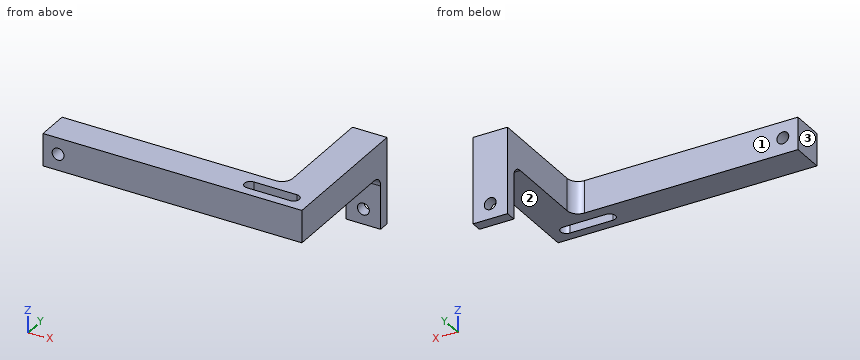
from build123d import *

# Parameters (mm, degrees)
BOSS_EXTRUDE1_DEPTH  = 15
SKETCH2_W            = 16
SKETCH2_H            = 5
BOSS_EXTRUDE2_DEPTH  = 40
CUT_EXTRUDE1_DEPTH   = 45
M5_CLEARANCE_HOLE1_D = 5.5
FILLET1_R            = 5


with BuildPart() as part:
    # Sketch1 → Boss-Extrude1 (new body)
    with BuildSketch(Plane.XY):
        Polygon((0, 0), (-120, 0), (-120, 15), (-16, 15), (-16, 62), (0, 62), align=None)
    extrude(amount=BOSS_EXTRUDE1_DEPTH)

    # Sketch2 → Boss-Extrude2 (add)
    with BuildSketch(Plane.XY.offset(15)):
        with Locations((-8, 64.5)):
            Rectangle(SKETCH2_W, SKETCH2_H)
    extrude(amount=-BOSS_EXTRUDE2_DEPTH)

    # Sketch3 → Cut-Extrude1 (cut)
    with BuildSketch(Plane.XY.offset(15)):
        with BuildLine():
            Line((-28, 9.7), (-8, 9.7))
            ThreePointArc((-8, 9.7), (-5.3, 7), (-8, 4.3))
            Line((-8, 4.3), (-28, 4.3))
            ThreePointArc((-28, 4.3), (-30.7, 7), (-28, 9.7))
        make_face()
    extrude(amount=-CUT_EXTRUDE1_DEPTH, mode=Mode.SUBTRACT)

    # M5 Clearance Hole1 (through all)
    with Locations(Plane(origin=(0, 67, 0), x_dir=(1, 0, 0), z_dir=(0, 1, 0))):
        with Locations((-8, 18), (-113, -7.5)):
            Hole(M5_CLEARANCE_HOLE1_D / 2)

    # Fillet1
    fillet1_edges = [part.edges().sort_by_distance(p)[0] for p in [
        (-16, 15, 7.5),
        (-8, 62, 0),
    ]]
    fillet(fillet1_edges, radius=FILLET1_R)


solid = part.part
Design review of the part built by this model. Coordinates are the model's own, in mm. Face numbers are marked on the shaded views. A direction names the side the tool comes from. Round coordinates to 2 decimals unless told otherwise and drop trailing zeros. Write each loop counter-clockwise with the first axis right and the second up, starting at its lowest first coordinate (ties: lowest second). Pieces come first, ordered by that corner, then holes. Notation, with made-up numbers: (56, -39.75) -> (68, -39.75) arc R17 cw to (68, -20.75) -> close; hole circle Ø8 at (87.5, 35). An arc over 180 degrees is marked (long way). One line per item, written item: value. Start each with the question number.
Q1. Tool access review of the marked faces 1, 2 and 3: name each direction out of +Z, -Z, +X, -X, +Y, -Y from which nothing blocks a thin tool from reaching the whole face with its end or side.
Q2. Add section D-D (z = -18). Give the boundary of the cut face in (x, y), then the cut area to 3 significant figures.
Q3. Add section B-B (y = 7). Give the boundary of the cut face in (x, z).
Q4. To check wall thickness, follow probe 1 along Z at (x, y) = (-8, 64); probe 2 along Y at (x, z) = (-12, 10.5); probe 3 along Z at (x, y) = (-113, 6.25). State the ranges of each line that lie inside material, in increasing order.
Q5. Add section A-A (z = 7.5). Give the boundary of the cut face in (x, y), then the cut area to 3 significant figures.
Q6. Add section C-C (x = -113). Give the boundary of the cut face in (y, z), then the cut area to 4 significant figures.
Q7. Insertion check: P1, Ø12, axis at x = -88, z = 10.5, coming from the +Y side; P2, Ø17.5, axis at x = -6, z = -15.5, coming from the -Y side. Each pin has a flat end and moves straight along its axis. Give the tip position at first contact, or say it passes through.
Response:
1. face 1: +Z, -Z, -X, +Y
1. face 2: -Z, +X, -X, -Y
1. face 3: +Z, -Z, -X, +Y, -Y
2. outline: (-16, 62) -> (-10.75, 62) -> (-10.75, 67) -> (-16, 67) -> close; (-5.25, 62) -> (0, 62) -> (0, 67) -> (-5.25, 67) -> close
2. area: 52.5 mm^2
3. outline: (-120, 0) -> (-30.7, 0) -> (-30.7, 15) -> (-120, 15) -> close; (-5.3, 0) -> (0, 0) -> (0, 15) -> (-5.3, 15) -> close; hole circle Ø5.5 at (-113, 7.5)
4. probe 1: z = -25 to -20.75, -15.25 to 15
4. probe 2: y = 0 to 4.3, 9.7 to 67
4. probe 3: z = 0 to 4.75, 10.25 to 15
5. outline: (-120, 0) -> (-115.75, 0) -> (-115.75, 15) -> (-120, 15) -> close; (-110.25, 0) -> (0, 0) -> (0, 67) -> (-16, 67) -> (-16, 20) arc R5 cw to (-21, 15) -> (-110.25, 15) -> close; hole (-28, 4.3) -> (-8, 4.3) arc R2.7 ccw to (-8, 9.7) -> (-28, 9.7) arc R2.7 ccw to start
5. area: 2,420 mm^2
6. outline: (0, 0) -> (15, 0) -> (15, 4.75) -> (0, 4.75) -> close; (0, 10.25) -> (15, 10.25) -> (15, 15) -> (0, 15) -> close
6. area: 142.5 mm^2
7. P1: stops at y = 15
7. P2: stops at y = 62
